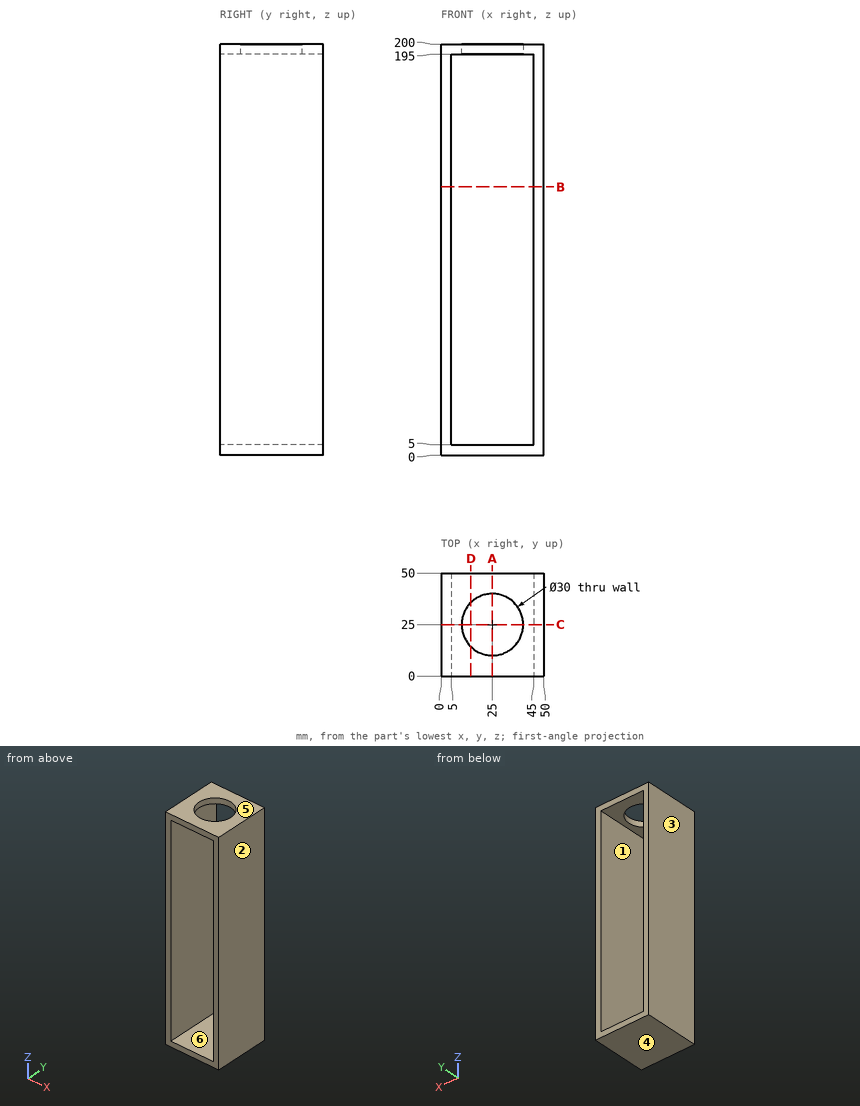
Geometry: see drawing. Coordinates: mm, zero at the bounding-box minimum. A direction names the side the tool comes from. Coordinates: 2 decimals unless noted, no trailing zeros. Loops run counter-clockwise (first coordinate to the right, second up) from the corner with the lowest first, then second, coordinate; pieces in that order, holes last. Notation, with made-up numbers: (21, 12.25) - (71, 12.25) arc R22 cw to (71, 29.25) - close; hole circle Ø7 at (58, 58). An arc over 180 degrees is marked (long way). Answer in a Markdown table with one row per item.
(1) Set-up query: the marked faces 5 and 6. Return all of +Z, -Z, +X, -X, +Y, -Y with unobstructed straight access to the full face (end or side cutting, diameter ignored); none if empty.
Model answer:
| item | result |
|---|---|
| face 5 | +Z, +X, -X, +Y, -Y |
| face 6 | +Y, -Y |
(2) Cut plane C-C on y = 25. Output: boundary loops of the cut face in (x, z).
Model answer:
| item | result |
|---|---|
| outline | (0, 0) - (50, 0) - (50, 200) - (40, 200) - (40, 195) - (45, 195) - (45, 5) - (5, 5) - (5, 195) - (10, 195) - (10, 200) - (0, 200) - close |
(3) Cut plane A-A on x = 25. Output: boundary loops of the cut face in (y, z).
Model answer:
| item | result |
|---|---|
| outline | (0, 0) - (50, 0) - (50, 5) - (0, 5) - close; (0, 195) - (10, 195) - (10, 200) - (0, 200) - close; (40, 195) - (50, 195) - (50, 200) - (40, 200) - close |
(4) Material intervals for L1, parallel to X at y = 33, z = 75; L2, parallel to Y at x = 25, z = 196.45; L3, parallel to Z at x = 38, y = 11, sorted ascending. Write a range as from..to.
Model answer:
| item | result |
|---|---|
| L1 | x = 0..5, 45..50 |
| L2 | y = 0..10, 40..50 |
| L3 | z = 0..5, 195..200 |
(5) Cut plane D-D on x = 14.5. Output: boundary loops of the cut face in (y, z), plus the area to 3 significant figures.
Model answer:
| item | result |
|---|---|
| outline | (0, 0) - (50, 0) - (50, 5) - (0, 5) - close; (0, 195) - (14.29, 195) - (14.29, 200) - (0, 200) - close; (35.71, 195) - (50, 195) - (50, 200) - (35.71, 200) - close |
| area | 393 mm² |
(6) Mould query, pull axis X, two halves, no side actions, for the marked faces 1, 2, 3 and 4. Classes: pulls with the +X half, pulls with the -X half, needs draft (parallel to the pull), parting line crosses it, or undercut.
Model answer:
| item | result |
|---|---|
| face 1 | undercut |
| face 2 | pulls with the +X half |
| face 3 | pulls with the -X half |
| face 4 | needs draft |
(7) Cut plane B-B on z = 130.5. Output: boundary loops of the cut face in (x, y).
Model answer:
| item | result |
|---|---|
| outline | (0, 0) - (5, 0) - (5, 50) - (0, 50) - close; (45, 0) - (50, 0) - (50, 50) - (45, 50) - close |
